Geometry check sheet. Reference: the model listing, model coordinates, mm. A direction names the side the tool comes from. Give positions to 0.01 mm unless a question says otherwise; leave off trailing zeros. Write each loop counter-clockwise with the first axis right and the second up, starting at its lowest first coordinate (ties: lowest second). Pieces come first, ordered by that corner, then holes. Notation, with made-up numbers: (71, 24) - (88, 24) arc R28 cw to (88, 47) - close; hole circle Ø2 at (-22.5, 13). An arc over 180 degrees is marked (long way). Write item = value, one per line. Start each with the question number.
(1) Section check A-A, the plane x = 14. Enter the section's corners in (y, z), plus the area to 3 significant figures.
(2) Depth check by flat-ended pin: pin 1 Ø1.8 at (x, y) = (0, -21.5) entering from -Z. Enter the tip coordinate at first touch or a pass-through.
(3) Access from +Z, -Z, +X, -X, +Y, -Y to the whole of each face (thin tool, end or side, straight path). Record for faces 1 (the flat face through (10, -22, 2)), 2 (the cylindrical face through (-19.43, 3.6, 2.54)), 3 (the flat face through (-20, -15, 2)).
(4) Section check D-D, the plane x = -7. Enter the section's corners in (y, z), plus the area to 3 significant figures.
(5) Thickness scan on L1, parallel to Y at x = 8, z = 2.5; L2, parallel to Y at x = -7, z = 2; L3, parallel to Y at x = -14.5, z = 4.45. Record the ranges inside material, lowest first.
(6) Section check B-B, the plane y = 21.5. Enter the section's corners in (x, z), plus the area to 3 significant figures.
(7) Section check C-C, the plane x = 0. Enter the section's corners in (y, z), plus the area to 3 significant figures.
```python
from build123d import *

# Parameters (mm, degrees)
ESQUISSE1_R        = 1.5
ESQUISSE1_W        = 5
ESQUISSE1_H        = 5
BOSS_EXTRU_1_DEPTH = 5
CONG_1_R           = 2


with BuildPart() as part:
    # Esquisse1 → Boss.-Extru.1 (new body)
    with BuildSketch(Plane.XY):
        with BuildLine():
            Line((-20, 27), (20, 27))
            Line((20, 27), (20, -27))
            Line((20, -27), (-20, -27))
            Line((-20, -27), (-20, -3))
            Line((-20, -3), (-5.196152423, -3))
            ThreePointArc((-5.196152423, -3), (6, 0), (-5.196152423, 3))
            Line((-5.196152423, 3), (-20, 3))
            Line((-20, 3), (-20, 27))
        make_face()
        with Locations((14, 0)):
            Circle(ESQUISSE1_R, mode=Mode.SUBTRACT)
        with Locations((-7, -12.124355653)):
            Circle(ESQUISSE1_R, mode=Mode.SUBTRACT)
        with Locations((-7, 12.124355653)):
            Circle(ESQUISSE1_R, mode=Mode.SUBTRACT)
        with Locations((0, 21.5)):
            Circle(ESQUISSE1_R, mode=Mode.SUBTRACT)
        with Locations(Location((0, -21.5, 0), (0, 0, 90))):
            Circle(ESQUISSE1_R, mode=Mode.SUBTRACT)
        with Locations((-7.5, 21.5)):
            Rectangle(ESQUISSE1_W, ESQUISSE1_H, mode=Mode.SUBTRACT)
        with Locations((7.5, 21.5)):
            Rectangle(ESQUISSE1_W, ESQUISSE1_H, mode=Mode.SUBTRACT)
        with Locations((-7.5, -21.5)):
            Rectangle(ESQUISSE1_W, ESQUISSE1_H, mode=Mode.SUBTRACT)
        with Locations((7.5, -21.5)):
            Rectangle(ESQUISSE1_W, ESQUISSE1_H, mode=Mode.SUBTRACT)
    extrude(amount=BOSS_EXTRU_1_DEPTH)

    # Congé1
    cong_1_edges = [part.edges().sort_by_distance(p)[0] for p in [
        (-20, -27, 2.5),
        (-20, -3, 2.5),
        (-5.196152423, -3, 2.5),
        (-5.196152423, 3, 2.5),
        (-20, 3, 2.5),
        (-20, 27, 2.5),
        (20, 27, 2.5),
        (20, -27, 2.5),
    ]]
    fillet(cong_1_edges, radius=CONG_1_R)


solid = part.part
```
Model answer:
q1.outline = (-27, 0) - (-1.5, 0) - (-1.5, 5) - (-27, 5) - close; (1.5, 0) - (27, 0) - (27, 5) - (1.5, 5) - close
q1.area = 255 mm²
q2.pin_1 = through
q3.face_1 = +Z, -Z
q3.face_2 = +Z, -Z, -X
q3.face_3 = +Z, -Z, -X, +Y, -Y
q4.outline = (-27, 0) - (-24, 0) - (-24, 5) - (-27, 5) - close; (-19, 0) - (-13.62, 0) - (-13.62, 5) - (-19, 5) - close; (-10.62, 0) - (-3, 0) - (-3, 5) - (-10.62, 5) - close; (3, 0) - (10.62, 0) - (10.62, 5) - (3, 5) - close; (13.62, 0) - (19, 0) - (19, 5) - (13.62, 5) - close; (24, 0) - (27, 0) - (27, 5) - (24, 5) - close
q4.area = 160 mm²
q5.L1 = -27 to -24, -19 to 19, 24 to 27
q5.L2 = -27 to -24, -19 to -13.62, -10.62 to -3, 3 to 10.62, 13.62 to 19, 24 to 27
q5.L3 = -27 to -3, 3 to 27
q6.outline = (-20, 0) - (-10, 0) - (-10, 5) - (-20, 5) - close; (-5, 0) - (-1.5, 0) - (-1.5, 5) - (-5, 5) - close; (1.5, 0) - (5, 0) - (5, 5) - (1.5, 5) - close; (10, 0) - (20, 0) - (20, 5) - (10, 5) - close
q6.area = 135 mm²
q7.outline = (-27, 0) - (-23, 0) - (-23, 5) - (-27, 5) - close; (-20, 0) - (-6, 0) - (-6, 5) - (-20, 5) - close; (6, 0) - (20, 0) - (20, 5) - (6, 5) - close; (23, 0) - (27, 0) - (27, 5) - (23, 5) - close
q7.area = 180 mm²
